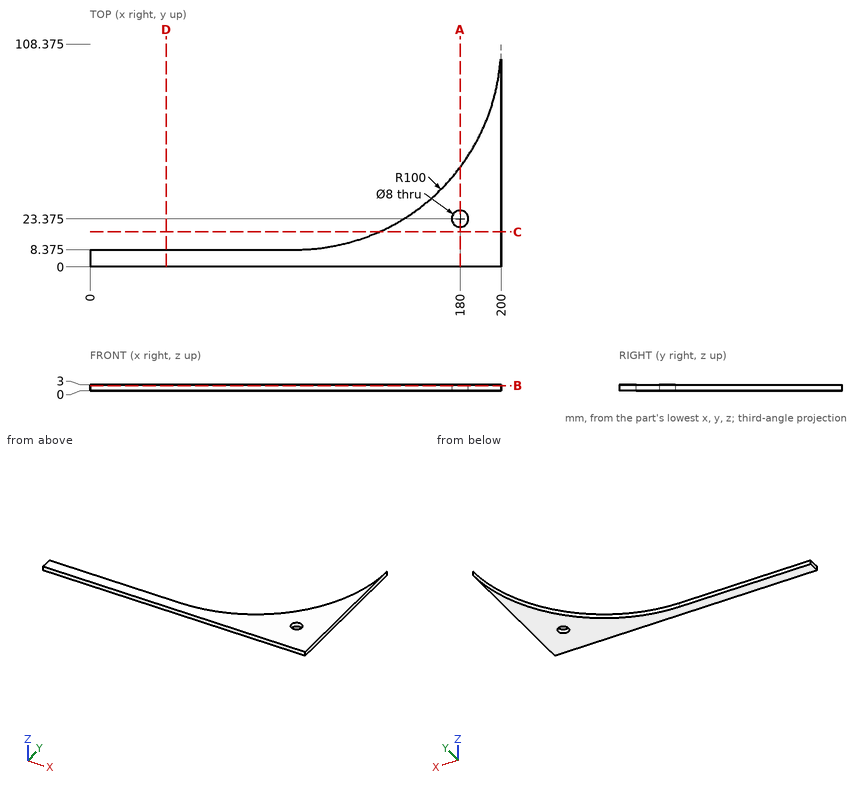
Can you work these out from the drawing? Everything is in mm from the part's minimum corner. Round coordinates to 2 decimals unless told otherwise and drop trailing zeros. Loops run counter-clockwise (first coordinate to the right, second up) from the corner with the lowest first, then second, coordinate; pieces in that order, holes last. Notation, with made-up numbers: (-3.75, 38) -> (35.25, 38) arc R25 cw to (35.25, 56) -> close; hole circle Ø6 at (1.25, -10.5). An arc over 180 degrees is marked (long way). Answer in a Markdown table with one row per item.
Item 1: If I drill on probe 1 along Y at (x, z) = (180, 1) (3 decimals); probe 2 along Y at (x, z) = (31.5, 1.5) (3 decimals); probe 3 along Y at (x, z) = (144, 0.5), over which ranges is the centre line in solid material (lowest first)?
Answer block:
| item | result |
|---|---|
| probe 1 | 0 to 19.375, 27.375 to 48.375 |
| probe 2 | 0 to 8.375 |
| probe 3 | 0 to 18.58 |
Item 2: Suppose I cut it at B-B, the plane z = 2.55. List the corners of the cut face in (x, y) for me (3 decimals), plus the area to 3 significant figures.
Answer block:
| item | result |
|---|---|
| outline | (0, 0) -> (200, 0) -> (200, 108.375) arc R100 cw to (100, 8.375) -> (0, 8.375) -> close; hole circle Ø8 at (180, 23.375) |
| area | 3,770 mm² |
Item 3: Will this pin go through, and if not, where does the flat tip stop? P1, Ø5, axis at x = 180, y = 23.375, coming from the -Z side.
Answer block:
| item | result |
|---|---|
| P1 | through |
Item 4: Suppose I cut it at D-D, the plane x = 37. List the corners of the cut face in (y, z) for me (3 decimals).
Answer block:
| item | result |
|---|---|
| outline | (0, 0) -> (8.375, 0) -> (8.375, 3) -> (0, 3) -> close |
Item 5: Suppose I cut it at C-C, the plane y = 17. List the corners of the cut face in (x, z) for me.
Answer block:
| item | result |
|---|---|
| outline | (140.63, 0) -> (200, 0) -> (200, 3) -> (140.63, 3) -> close |
Item 6: Suppose I cut it at A-A, the plane x = 180. List the corners of the cut face in (y, z) for me (3 decimals).
Answer block:
| item | result |
|---|---|
| outline | (0, 0) -> (19.375, 0) -> (19.375, 3) -> (0, 3) -> close; (27.375, 0) -> (48.375, 0) -> (48.375, 3) -> (27.375, 3) -> close |
